```python
from build123d import *
from OCP.BRepFilletAPI import BRepFilletAPI_MakeChamfer

# Parameters (mm, degrees)
BOSS_EXTRUDE1_DEPTH = 27.432
CHAMFER1_SIZE       = 0.254
CHAMFER1_SIZE2      = 0.146646968


# Read off the part's stored shape, not the designer's step: Cut-Revolve4
with BuildPart() as part:
    # Sketch3 → Boss-Extrude1 (new body)
    with BuildSketch(Plane(origin=(0, 0, 0), x_dir=(1, 0, 0), z_dir=(0, 1, 0))):
        Polygon((4.7625, 2.749630657), (0, 5.499261314), (-4.7625, 2.749630657), (-4.7625, -2.749630657), (0, -5.499261314), (4.7625, -2.749630657), align=None)
    extrude(amount=BOSS_EXTRUDE1_DEPTH)

    # Cut-Revolve4 outline → Cut-Revolve4 (revolve, cut)
    with BuildSketch(Plane.XY):
        Polygon((4.6609, 9.18188181), (3.1369, 8.302), (5.499261314, 8.302), (5.499261314, 27.432), (2.54, 27.432), (2.54, 16.302), (3.1369, 16.302), (4.6609, 15.42211819), align=None)
        Polygon((0.99695, 21.082), (2, 21.082), (2, 27.432), (0, 27.432), (0, 1.391072642), (0.99695, 1.92116036), align=None)
    revolve(axis=Axis((0, 0, 0), (0, 1, 0)), mode=Mode.SUBTRACT)

    # Chamfer1: one chamfer whose edges measure the first distance from different faces: ONE call of the kernel's chamfer builder (chamfer() names one face for all edges)
    chamfer1_edges_1 = [part.edges().sort_by_distance(p)[0] for p in [
        (-2.54, 27.432, 0),
    ]]
    chamfer1_side_1 = [part.faces().sort_by_distance(p)[0] for p in [
        (-2.468157951, 27.432, 0),
    ]]
    chamfer1_edges_2 = [part.edges().sort_by_distance(p)[0] for p in [
        (-2, 27.432, 0),
    ]]
    chamfer1_side_2 = [part.faces().sort_by_distance(p)[0] for p in [
        (-2, 24.257, 0),
    ]]
    chamfer1 = BRepFilletAPI_MakeChamfer(part.part.solid().wrapped)
    for e in chamfer1_edges_1:
        chamfer1.Add(CHAMFER1_SIZE, CHAMFER1_SIZE2, e.wrapped, chamfer1_side_1[0].wrapped)  # the first distance lies on this face
    for e in chamfer1_edges_2:
        chamfer1.Add(CHAMFER1_SIZE, CHAMFER1_SIZE2, e.wrapped, chamfer1_side_2[0].wrapped)  # the first distance lies on this face
    add(Compound.cast(chamfer1.Shape()), mode=Mode.REPLACE)

    # Sketch4 → Cut-Revolve5 (revolve, cut)
    with BuildSketch(Plane.XY, mode=Mode.PRIVATE) as cut_revolve5_sk:
        Polygon((-0.175, 0.762), (-0.5, 0.762), (-3, 2.091273579), (-3, 5.762), (-6.107414125, 5.762), (-6.107414125, 0), (0, 0), (0, 1.524), (-0.175, 1.524), align=None)
    revolve(cut_revolve5_sk.sketch.rotate(Axis((0, 0, 0), (0, 1, 0)), 270), axis=Axis((0, 0, 0), (0, 1, 0)), mode=Mode.SUBTRACT)


solid = part.part
```
Work out the finished part from the listing and answer in its coordinate system (mm). A direction names the side the tool comes from. Give positions to 0.01 mm unless a question says otherwise; leave off trailing zeros. Order: outer loops, then holes, each group sorted by start corner. A loop starts at its lowest first (then second) coordinate and runs counter-clockwise, first axis right, second up. Notation, with made-up numbers: M -7,81 L 46,81 A8 ccw 46,95 Z; hole C 10.25,10.25 d3. An arc over 180 degrees is marked long. Return JSON: item names as keys, results as strings.
1) A tool of negligible diameter and unlimited length cuts with its end or side. For faces 5 (the flat face through (3.24, 8.302, 1.15)), 6 (the cylindrical face through (-0.9, 3.95, -2.86)), 7 (the flat face through (-2.41, 7.01, 4.11)), 8 (the flat face through (-1, 21.082, 1)), 9 (the flat face through (2.348, 7.014, 4.144)), from which of +Z, -Z, +X, -X, +Y, -Y can it reach the whole face along a straight path? Write none if from no direction.
Resolved:
{"face 5": "none", "face 6": "-Y", "face 7": "+Z, -X, +Y, -Y", "face 8": "+Y", "face 9": "+Z, +X, +Y, -Y"}
2) Section B-B, the plane y = 22 is taken. Write down the section's boundary in (x, z), plus the area to 3 significant figures.
Resolved:
{"outline": "C 0,0 d5.08; hole C 0,0 d4", "area": "7.70 mm^2"}
3) Straight lines are drawn through the part: line 1 along Z through (x, y) = (0, 12.75); line 2 along Z through (x, y) = (0, 23). For each, find the intervals that lie inside material, in ascending order. Write a range as [from, to].
Resolved:
{"line 1": "[-4.66, -1], [1, 4.66]", "line 2": "[-2.54, -2], [2, 2.54]"}
4) For a pull along X with two mould halves and no side action, classify faces 1 (the flat face through (-4.762, 7, 0)), 2 (the cylindrical face through (-0.33, 21.72, -2.52)), 3 (the cylindrical face through (0.95, 11.64, -0.3)), 4 (the cylindrical face through (0, 24, 2)) as +X half, -X half, draft (parallel to the pull), parting line (faces both ways), or undercut.
Resolved:
{"face 1": "-X half", "face 2": "parting line", "face 3": "undercut", "face 4": "undercut"}
5) Each of these flat-tipped pins is pushed along its axis until it touches: pin 1 (5 mm diameter, centred on y = 7, z = -3.5, fed in from +X); pin 2 (2.5 mm diameter, centred on x = 0, z = 0, fed in from +Y); pin 3 (4 mm diameter, centred on y = 20.5, z = 1.5, fed in from +X); pin 4 (1 mm diameter, centred on y = 11.5, z = -0.5, fed in from +X). Where does it stop, or does it pass through?
Resolved:
{"pin 1": "x = 4.76", "pin 2": "y = 21.08", "pin 3": "x = 2.54", "pin 4": "x = 4.66"}
6) Section A-A, the plane y = 19 is taken. Write down the section's boundary in (x, z).
Resolved:
{"outline": "C 0,0 d5.08; hole C 0,0 d1.99"}
